from build123d import *

# Parameters (mm, degrees)
SKETCH1_W           = 12
SKETCH1_H           = 10
BOSS_EXTRUDE1_DEPTH = 15
FILLET1_R           = 4
SKETCH3_W           = 12
SKETCH3_H           = 10
BOSS_EXTRUDE2_DEPTH = 12.5
SKETCH4_R           = 2
BOSS_EXTRUDE3_DEPTH = 0.7
BOSS_EXTRUDE4_DEPTH = 9.3
SKETCH7_R           = 0.8
CUT_EXTRUDE1_DEPTH  = 2
BOSS_EXTRUDE5_START = 1.2
SKETCH8_R           = 2
BOSS_EXTRUDE5_DEPTH = 1.2
FILLET2_R           = 0.5


with BuildPart() as part:
    # Sketch1 → Boss-Extrude1 (new body)
    with BuildSketch(Plane.XY):
        with Locations((6, 5)):
            Rectangle(SKETCH1_W, SKETCH1_H)
    extrude(amount=BOSS_EXTRUDE1_DEPTH)

    # Fillet1
    fillet1_edges = [part.edges().sort_by_distance(p)[0] for p in [
        (0, 10, 7.5),
        (12, 10, 7.5),
        (12, 0, 7.5),
        (0, 0, 7.5),
    ]]
    fillet(fillet1_edges, radius=FILLET1_R)

    # Sketch3 → Boss-Extrude2 (add)
    with BuildSketch(Plane.XY):
        with Locations((6, 5)):
            Rectangle(SKETCH3_W, SKETCH3_H)
    extrude(amount=-BOSS_EXTRUDE2_DEPTH)

    # Sketch4 → Boss-Extrude3 (add)
    with BuildSketch(Plane(origin=(0, 0, -12.5), x_dir=(-1, 0, 0), z_dir=(0, 0, -1))):
        with Locations((-6, 5)):
            Circle(SKETCH4_R)
    extrude(amount=BOSS_EXTRUDE3_DEPTH)

    # Sketch5 → Boss-Extrude4 (add)
    with BuildSketch(Plane(origin=(0, 0, -13.2), x_dir=(-1, 0, 0), z_dir=(0, 0, -1))):
        with BuildLine():
            Line((-7.118033989, 6), (-4.881966011, 6))
            ThreePointArc((-4.881966011, 6), (-6, 3.5), (-7.118033989, 6))
        make_face()
    extrude(amount=BOSS_EXTRUDE4_DEPTH)

    # Sketch7 → Cut-Extrude1 (cut)
    with BuildSketch(Plane(origin=(0, 0, -12.5), x_dir=(-1, 0, 0), z_dir=(0, 0, -1))):
        with Locations((-10.5, 5)):
            Circle(SKETCH7_R)
        with Locations((-1.5, 5)):
            Circle(SKETCH7_R)
    extrude(amount=-CUT_EXTRUDE1_DEPTH, mode=Mode.SUBTRACT)

    # Sketch8 → Boss-Extrude5 (add)
    with BuildSketch(Plane.XY.offset(15).offset(BOSS_EXTRUDE5_START)):
        with Locations(Location((6, 5, 0), (0, 0, 180))):
            Circle(SKETCH8_R)
    extrude(amount=-BOSS_EXTRUDE5_DEPTH)

    # Fillet2
    fillet2_edges = [part.edges().sort_by_distance(p)[0] for p in [
        (0, 0, -6.25),
        (0, 10, -6.25),
        (12, 10, -6.25),
        (12, 0, -6.25),
    ]]
    fillet(fillet2_edges, radius=FILLET2_R)


solid = part.part
CAD build for the part. Positions are in the model's coordinates, mm. A direction names the side the tool comes from. Give positions to 0.01 mm unless a question says otherwise; leave off trailing zeros. Loops run counter-clockwise (first coordinate to the right, second up) from the corner with the lowest first, then second, coordinate; pieces in that order, holes last. Notation, with made-up numbers: M -17,-8.5 L 23,-8.5 A17 ccw 23,21.5 Z; hole C 39,-11.75 d7. An arc over 180 degrees is marked long. Answer in a Markdown table with one row per item. Add a question column.
Item 1: Band-saw the part on A-A on z = 5. Give the cut face in (x, y), then the cut area to 3 significant figures.
Item 2: Drop flat-ended pins along their axis: P1, Ø0.8, axis at x = 10.5, y = 5.5, coming from the -Z side; P2, Ø1.5, axis at x = 2.5, y = 2, coming from the +Z side; P3, Ø3, axis at y = 2.5, z = 8.5, coming from the -X side; P4, Ø1, axis at x = 1.5, y = 5, coming from the -Z side. Give the stop position or say it passes through.
Item 3: Probe probe 1 along Y at (x, z) = (10.5, -11.35); probe 2 along Z at (x, y) = (9.5, 8.25); probe 3 along Z at (x, y) = (11, 4.5). List the from-to ranges inside material, lowest first.
Item 4: Tool access for faces 5 (the face through (10.859, 8.797, 7.605)), 6 (the face through (6, 6, -18)), 7 (the face through (6, 6.4, -13.2)): list every direction of +Z, -Z, +X, -X, +Y, -Y with a clear straight run to the whole face (end or side of a thin tool).
Item 5: Band-saw the part on D-D on y = 1.5. Give the cut face in (x, z), then the cut area to 3 significant figures.
Item 6: Band-saw the part on C-C on x = 6. Give the cut face in (y, z).
Item 7: Band-saw the part on B-B on y = 5. Give the cut face in (x, z), then the cut area to 3 significant figures.
Item 8: Mould opens along X. For faces 1 (the face through (1.67, 4.22, -11.51)), 2 (the face through (11, 5, -10.5)), 3 (the face through (0, 5, -5)), 4 (the face through (6, 10, -2)) say: +X half, -X half, draft (parallel to the pull), parting line (faces both ways), or undercut.
Reply:
| question | item | result |
|---|---|---|
| 1 | outline | M 0,4 A4 ccw 4,0 L 8,0 A4 ccw 12,4 L 12,6 A4 ccw 8,10 L 4,10 A4 ccw 0,6 Z |
| 1 | area | 106 mm^2 |
| 2 | P1 | stops at z = -12.5 |
| 2 | P2 | stops at z = 15 |
| 2 | P3 | stops at x = 0 |
| 2 | P4 | stops at z = -10.5 |
| 3 | probe 1 | y = 0 to 4.2, 5.8 to 10 |
| 3 | probe 2 | z = -12.5 to 15 |
| 3 | probe 3 | z = -10.5 to 15 |
| 4 | face 5 | +Z, +X, +Y |
| 4 | face 6 | -Z, +X, -X, +Y |
| 4 | face 7 | -Z |
| 5 | outline | M 0,-12.5 L 12,-12.5 L 12,0 L 11.12,0 L 11.12,15 L 0.88,15 L 0.88,0 L 0,0 Z |
| 5 | area | 304 mm^2 |
| 6 | outline | M 0,-12.5 L 3,-12.5 L 3,-13.2 L 3.5,-13.2 L 3.5,-22.5 L 6,-22.5 L 6,-13.2 L 7,-13.2 L 7,-12.5 L 10,-12.5 L 10,15 L 7,15 L 7,16.2 L 3,16.2 L 3,15 L 0,15 Z |
| 7 | outline | M 0,-12.5 L 0.7,-12.5 L 0.7,-10.5 L 2.3,-10.5 L 2.3,-12.5 L 4,-12.5 L 4,-13.2 L 4.5,-13.2 L 4.5,-22.5 L 7.5,-22.5 L 7.5,-13.2 L 8,-13.2 L 8,-12.5 L 9.7,-12.5 L 9.7,-10.5 L 11.3,-10.5 L 11.3,-12.5 L 12,-12.5 L 12,15 L 8,15 L 8,16.2 L 4,16.2 L 4,15 L 0,15 Z |
| 7 | area | 359 mm^2 |
| 8 | face 1 | undercut |
| 8 | face 2 | undercut |
| 8 | face 3 | -X half |
| 8 | face 4 | draft |
